Autodesk Inventor part; units mm, degrees
ref_plane "РабПлоскость1" through (22.5, 0, 17.5) normal (1, 0, 0) x (0, 0, -1)
ref_plane "YZ Plane" through (0, 0, 0) normal (1, 0, 0) x (0, 1, 0)
ref_plane "XZ Plane" through (0, 0, 0) normal (0, 1, 0) x (-1, 0, 0)
sketch "Эскиз1" plane through (0, 0, 0) normal (1, 0, 0) x (0, 1, 0)
  line L0 (-6, -6.0208) -> (-6, 6.0208)
  arc A0 (-6, -6.0208) -> (6, -6.0208) centre (0, 0) ccw
  line L1 (6, 6.0208) -> (6, -6.0208)
  arc A1 (6, 6.0208) -> (-6, 6.0208) centre (0, 0) ccw
  circle A2 centre (0, 0) radius 17.5
  line L2 (0, 17.5) -> (80, 17.5)
  line L3 (80, 17.5) -> (80, -17.5)
  line L4 (80, -17.5) -> (0, -17.5)
  line L5 (0, -17.5) -> (0, -8.5)
  line L6 (0, 8.5) -> (0, 17.5)
  dimension "d0" = 35
  dimension "d1" = 80
extrude "Выдавливание1" add sketch "Эскиз1" along normal blind 45 contours A0 L5 A2 L6 A1 L0 | A0 L1 A1 L6 A2 L5 | A2 L2 L3 L4
sketch "Эскиз2" plane through (45, 0, 0) normal (1, 0, 0) x (0, 0, -1)
  line L0 (17.5, 80) -> (-17.5, 80)
  line L1 (17.5, 0) -> (17.5, 80)
  line L2 (-17.5, 80) -> (17.5, 80)
  line L3 (17.5, 80) -> (17.5, 57)
  line L4 (17.5, 57) -> (-17.5, 57)
  line L5 (-17.5, 57) -> (-17.5, 80)
  point P0 (0, 0)
  dimension "d4" = 23
extrude "Выдавливание2" add sketch "Эскиз2" along normal blind 22
ref_plane "РабПлоскость1" through (22.5, 0, 17.5) normal (1, 0, 0) x (0, 0, -1)
mirror "Зеркальное отражение1" about plane through (22.5, 0, 17.5) normal (1, 0, 0) of "Выдавливание2"
sketch "Эскиз3" plane through (45, 0, 0) normal (1, 0, 0) x (0, 0, -1)
  arc A0 (6.0208, -6) -> (6.0208, 6) centre (0, 0) ccw
  line L0 (6.0208, -6) -> (-6.0208, -6)
  arc A1 (-6.0208, 6) -> (-6.0208, -6) centre (0, 0) ccw
  line L1 (6.0208, 6) -> (-6.0208, 6)
  line L2 (17.5, 57) -> (-17.5, 57)
  line L3 (-17.5, 57) -> (-17.5, 0)
  arc A2 (-17.5, 0) -> (17.5, 0) centre (0, 0) ccw
  line L4 (17.5, 0) -> (17.5, 57)
sketch "Эскиз4" plane through (67, 0, 0) normal (1, 0, 0) x (0, 0, -1)
  arc A0 (6.0208, -6) -> (6.0208, 6) centre (0, 0) ccw
  line L0 (6.0208, -6) -> (-6.0208, -6)
  arc A1 (-6.0208, 6) -> (-6.0208, -6) centre (0, 0) ccw
  line L1 (6.0208, 6) -> (-6.0208, 6)
  line L2 (17.5, 37) -> (-17.5, 37)
  line L3 (-17.5, 37) -> (-17.5, 0)
  arc A2 (-17.5, 0) -> (17.5, 0) centre (0, 0) ccw
  line L4 (17.5, 0) -> (17.5, 37)
  line L5 (17.5, 0) -> (17.5, 57)
  line L6 (-17.5, 37) -> (17.5, 37)
  line L7 (17.5, 37) -> (17.5, 57)
  line L8 (17.5, 57) -> (-17.5, 57)
  line L9 (-17.5, 57) -> (-17.5, 37)
extrude "Выдавливание3" add sketch "Эскиз4" against normal blind 8
mirror "Зеркальное отражение2" about plane through (22.5, 0, 17.5) normal (1, 0, 0) of "Выдавливание3"
sketch "Эскиз5" plane through (67, 80, 17.5) normal (0, 1, 0) x (1, 0, 0)
  line L0 (-89, 35) -> (-89, 0)
  line L1 (-89, 35.1034) -> (-89, 0)
  line L2 (-89, 0) -> (-89, 35.1034)
  line L3 (-89, 35) -> (0, 35)
  line L4 (-89, 35) -> (0, 35)
  line L5 (-89, 17.5517) -> (-44.5, 17.5517)
  circle A0 centre (-44.5, 17.5517) radius 4.1
  line L6 (-44.5, 17.5517) -> (-59.5, 17.5517)
  circle A1 centre (-59.5, 17.5517) radius 7.5
  line L7 (-44.5, 17.5517) -> (-29.5, 17.5517)
  circle A2 centre (-29.5, 17.5517) radius 7.5
  point P0 (-67, 17.5)
  dimension "d9" = 8.2
  dimension "d10" = 15
  dimension "d11" = 15
  dimension "d12" = 15
  dimension "d13" = 15
extrude "Выдавливание4" add sketch "Эскиз5" along normal blind 10 contours L5 A1 | L5 A1 | A2
sketch "Эскиз6" plane through (67, 80, 17.5) normal (0, 1, 0) x (1, 0, 0)
  line L0 (-89, 35) -> (-89, 0)
  line L1 (-89, 35.1034) -> (-89, 0)
  line L2 (-89, 0) -> (-89, 35.1034)
  line L3 (-89, 35) -> (0, 35)
  line L4 (-89, 35) -> (0, 35)
  line L5 (-89, 17.5517) -> (-44.5, 17.5517)
  circle A0 centre (-44.5, 17.5517) radius 4.1
  line L6 (-44.5, 17.5517) -> (-59.5, 17.5517)
  circle A1 centre (-59.5, 17.5517) radius 7.5
  line L7 (-44.5, 17.5517) -> (-29.5, 17.5517)
  circle A2 centre (-29.5, 17.5517) radius 7.5
  point P0 (-67, 17.5)
  point P1 (-67, 17.5)
  dimension "d16" = 8.2
  dimension "d17" = 15
  dimension "d18" = 15
  dimension "d19" = 15
  dimension "d20" = 15
extrude "Выдавливание5" cut sketch "Эскиз6" against normal blind 35 contours A0 L7 L5 | L5 L7 A0
sketch "Эскиз7" plane through (0, 0, 17.5) normal (0, 0, 1) x (1, 0, 0)
  line L0 (18.4, 80) -> (18.4, 45)
  line L1 (26.6, 80) -> (26.6, 45)
  line L2 (0, 57) -> (0, 0)
  line L3 (45, 0) -> (0, 0)
  line L4 (45, 57) -> (45, 0)
  line L5 (45, 57) -> (59, 57)
  line L6 (67, 80) -> (67, 0)
  line L7 (-22, 80) -> (67, 80)
  line L8 (-22, 80) -> (-22, 0)
  line L9 (0, 57) -> (-14, 57)
  line L10 (18.4, 45) -> (26.6, 45)
  line L11 (18.4, 45) -> (8.4, 45)
  line L12 (8.4, 45) -> (8.4, 55)
  line L13 (8.4, 55) -> (36.6, 55)
  line L14 (36.6, 55) -> (36.6, 45)
  line L15 (26.6, 45) -> (36.6, 45)
  line L16 (18.4, 45) -> (26.6, 45)
  line L17 (59, 0) -> (59, 57)
  line L18 (67, 0) -> (59, 0)
  line L19 (-22, 0) -> (-14, 0)
  line L20 (-14, 0) -> (-14, 57)
  dimension "d23" = 10
  dimension "d24" = 10
  dimension "d25" = 28.2
  dimension "d26" = 10
extrude "Выдавливание6" cut sketch "Эскиз7" against normal blind 84.5 contours L13 L1 L10 L0 | L0 L11 L12 L13 | L13 L14 L15 L1
sketch "Эскиз8" plane through (0, 0, 17.5) normal (0, 0, 1) x (1, 0, 0)
  line L0 (8.4, 45) -> (36.6, 45)
  line L1 (8.4, 45) -> (0, 45)
  line L2 (0, 45) -> (0, 36)
  line L3 (0, 0) -> (0, 57)
  line L4 (45, -17.5) -> (45, 0)
  line L5 (0, 36) -> (45, 36)
  line L6 (45, 36) -> (45, -17.5)
  line L7 (45, -17.5) -> (0, -17.5)
  line L8 (0, -17.5) -> (0, 36)
  dimension "d29" = 9
extrude "Выдавливание7" cut sketch "Эскиз8" against normal blind 85.25
sketch "Эскиз9" plane through (67, 0, 0) normal (1, 0, 0) x (0, 0, -1)
  circle A0 centre (0, 0) radius 11.4
  dimension "d32" = 22.8
extrude "Выдавливание8" cut sketch "Эскиз9" against normal blind 144.5
sketch "Эскиз10" plane through (-22, 80, 17.5) normal (0, 0, 1) x (1, 0, 0)
  line L0 (22, -23) -> (22, -44)
  line L1 (67, -23) -> (67, -44)
  line L2 (22, -44) -> (67, -44)
  line L3 (67, -44) -> (67, -35)
  line L4 (67, -35) -> (22, -35)
  line L5 (22, -35) -> (22, -44)
  point P0 (22, -80)
  dimension "d35" = 9
extrude "Выдавливание9" add sketch "Эскиз10" along normal blind 45
sketch "Эскиз11" plane through (67, 45, 17.5) normal (0, 1, 0) x (1, 0, 0)
  line L0 (-67, 0) -> (-67, 35)
  line L1 (-67, 0) -> (-44.5, 0)
  line L2 (-67, 0) -> (-58.6, 0)
  line L3 (-22, -45) -> (-67, -45)
  line L4 (-44.5, -45) -> (-44.5, -21)
  line L5 (-27, -42) -> (-23.5, -38.5)
  line L6 (-23.5, -38.5) -> (-23.5, -3.5)
  line L7 (-23.5, -3.5) -> (-27, 0)
  line L8 (-27, 0) -> (-62, 0)
  line L9 (-62, 0) -> (-65.5, -3.5)
  line L10 (-65.5, -3.5) -> (-65.5, -38.5)
  line L11 (-65.5, -38.5) -> (-62, -42)
  line L12 (-62, -42) -> (-27, -42)
  circle A0 centre (-44.5, -21) radius 11.3
  circle A1 centre (-29, -5.5) radius 1.25
  circle A2 centre (-60, -5.5) radius 1.25
  circle A3 centre (-60, -36.5) radius 1.25
  circle A4 centre (-29, -36.5) radius 1.25
  line L13 (-52.5, -48) -> (-50.5, -48)
  line L14 (-50.5, -41.8) -> (-50.5, -48)
  line L15 (-57.9172, -41.8) -> (-50.5, -41.8)
  line L16 (-65.3, -34.4172) -> (-57.9172, -41.8)
  line L17 (-65.3, -7.5828) -> (-65.3, -34.4172)
  line L18 (-57.9172, -0.2) -> (-65.3, -7.5828)
  line L19 (-31.0828, -0.2) -> (-57.9172, -0.2)
  line L20 (-23.7, -7.5828) -> (-31.0828, -0.2)
  line L21 (-23.7, -34.4172) -> (-23.7, -7.5828)
  line L22 (-31.0828, -41.8) -> (-23.7, -34.4172)
  line L23 (-38.5, -41.8) -> (-31.0828, -41.8)
  line L24 (-38.5, -41.8) -> (-38.5, -48)
  line L25 (-38.5, -48) -> (-36.5, -48)
  line L26 (-36.5, -48) -> (-36.5, -42)
  line L27 (-36.5, -42) -> (-27, -42)
  line L28 (-27, -42) -> (-23.5, -38.5)
  line L29 (-23.5, -38.5) -> (-23.5, -3.5)
  line L30 (-23.5, -3.5) -> (-27, 0)
  line L31 (-27, 0) -> (-62, 0)
  line L32 (-62, 0) -> (-65.5, -3.5)
  line L33 (-65.5, -3.5) -> (-65.5, -38.5)
  line L34 (-65.5, -38.5) -> (-62, -42)
  line L35 (-62, -42) -> (-52.5, -42)
  line L36 (-52.5, -42) -> (-52.5, -48)
  point P0 (-67, 17.5)
  dimension "d38" = 22.5
  dimension "d39" = 24
extrude "Выдавливание10" cut sketch "Эскиз11" against normal blind 45 contours A0 | A1 | A2 | A3 | A4
chamfer "Фаска1" distance 2 angle 45 4 edges at (5.75, 36, 54) (5.75, 36, 23) (36.75, 36, 23) (36.75, 36, 54)
chamfer "Фаска2" distance 6 angle 45 2 edges at (0, 40.5, 62.5) (45, 40.5, 62.5)
sketch "Эскиз13" plane through (-22, 80, 17.5) normal (0, 0, 1) x (1, 0, 0)
  line L0 (81, -80) -> (81, -23)
  line L1 (22, -23) -> (8, -23)
  line L2 (81, -44) -> (8, -44)
  line L3 (8, -44) -> (8, -23)
  line L4 (8, -23) -> (81, -23)
  line L5 (81, -23) -> (81, -44)
  line L6 (61, -44) -> (67, -44)
  line L7 (22, -35) -> (30.4, -35)
  line L8 (30.4, -25) -> (58.6, -25)
  line L9 (30.4, -35) -> (58.6, -35)
  line L10 (58.6, -35) -> (58.6, -25)
  line L11 (58.6, -25) -> (30.4, -25)
  line L12 (30.4, -25) -> (30.4, -35)
  point P0 (22, -80)
  dimension "d51" = 0
extrude "Выдавливание12" add sketch "Эскиз13" against normal up to surface (35 mm away)
properties part number "joint1_level_part_2" material "Пластик АБС"
Source: CAD feature listing. Evaluate the final solid. Frame: model axes, mm. A direction names the side the tool comes from. Round coordinates to 2 decimals unless told otherwise and drop trailing zeros. Loops run counter-clockwise (first coordinate to the right, second up) from the corner with the lowest first, then second, coordinate; pieces in that order, holes last.
Q1. Mould query, pull axis Y, two halves, no side actions, for faces 4 (the face through (-18, -7, 9)), 5 (the face through (7, 90, 0)), 6 (the face through (8.4, 50, 0)), 7 (the face through (59, 16, 0)). Classes: pulls with the +Y half, pulls with the -Y half, needs draft (parallel to the pull), parting line crosses it, or undercut.
Q2. Section A-A, the plane z = 2. State how many separate pieces and enclosed holes the cut face has, plus the area to 3 significant figures.
Q3. Section B-B, the plane x = 22. Return loops of the section in (y, z).
Q4. First-contact query: P1, Ø5, axis at x = 1.5, z = -6.5, coming from the -Y side; P2, Ø4, axis at x = 7.5, z = 37.5, coming from the +Y side; P3, Ø1.5, axis at x = 38, z = 54, coming from the -Y side; P4, Ø1, axis at x = 57.5, y = 50.5, coming from the +Z side. Flat tips, straight axial feed; report the tip coordinate or a pass-through.
Q5. Ray query, line 1 (X direction, y = 41.25, z = 23); line 2 (Z direction, x = 38, y = 40); line 3 (Z direction, x = 22.5, y = 72.5). Return the intervals inside material, ascending.
Q6. Access query for faces 1 (the face through (30, 85, 0)), 2 (the face through (36.6, 50, 0)), 3 (the face through (6.84, 41.55, 52.76)). Directions: +Z, -Z, +X, -X, +Y, -Y. A direction counts if a zero-diameter tool reaches every point of the face in a straight line with its end or side. Return the directions, or none.
Solutions:
1. face 4: undercut
1. face 5: pulls with the +Y half
1. face 6: undercut
1. face 7: needs draft
2. separate pieces: 3
2. enclosed holes: 1
2. area: 4,250 mm2
3. outline: (36, -17.5) - (45, -17.5) - (45, 27.21) - (36, 27.21) - close; (36, 49.79) - (45, 49.79) - (45, 62.5) - (36, 62.5) - close; (55, -17.5) - (80, -17.5) - (80, -4.12) - (57, -4.12) - (57, 4.02) - (80, 4.02) - (80, 17.5) - (55, 17.5) - close
4. P1: stops at y = 36
4. P2: stops at y = 45
4. P3: passes through
4. P4: stops at z = 17.5
5. line 1: x = 0 to 5.75, 8.25 to 36.75, 39.25 to 45
5. line 2: z = -17.5 to 21.75, 24.25 to 52.75, 55.25 to 62.5
5. line 3: z = -17.5 to -4.15, 4.05 to 17.5
6. face 1: +Y
6. face 2: +Z, -Z
6. face 3: +Y, -Y
